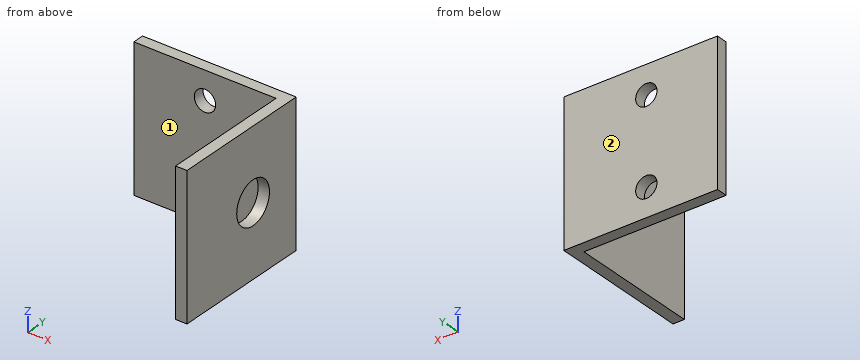
```python
from build123d import *

# Parameters (mm, degrees)
SKETCH2_W           = 20
SKETCH2_H           = 20
BOSS_EXTRUDE1_DEPTH = 1.6
SKETCH2_4_W         = 1.6
SKETCH2_4_H         = 20
BOSS_EXTRUDE2_DEPTH = 20
SKETCH3_R           = 3
CUT_EXTRUDE1_DEPTH  = 3
SKETCH4_R           = 1.5
CUT_EXTRUDE2_DEPTH  = 2


with BuildPart() as part:
    # Sketch2 → Boss-Extrude1 (new body)
    with BuildSketch(Plane(origin=(0, 0, 0), x_dir=(1, 0, 0), z_dir=(0, 1, 0))):
        Rectangle(SKETCH2_W, SKETCH2_H)
    extrude(amount=-BOSS_EXTRUDE1_DEPTH)

    # Sketch2_4 → Boss-Extrude2 (add)
    with BuildSketch(Plane(origin=(0, 0, 0), x_dir=(1, 0, 0), z_dir=(0, 1, 0))):
        with Locations((10.8, 0)):
            Rectangle(SKETCH2_4_W, SKETCH2_4_H)
    extrude(amount=-BOSS_EXTRUDE2_DEPTH)

    # Sketch3 → Cut-Extrude1 (cut)
    with BuildSketch(Plane(origin=(11.6, 0, 0), x_dir=(0, 0, -1), z_dir=(1, 0, 0))):
        with Locations((0, -7.888677581)):
            Circle(SKETCH3_R)
    extrude(amount=-CUT_EXTRUDE1_DEPTH, mode=Mode.SUBTRACT)

    # Sketch4 → Cut-Extrude2 (cut)
    with BuildSketch(Plane(origin=(0, 0, 0), x_dir=(1, 0, 0), z_dir=(0, 1, 0))):
        with Locations(Location((0, 6, 0), (0, 0, 270))):
            Circle(SKETCH4_R)
        with Locations(Location((0, -6, 0), (0, 0, 270))):
            Circle(SKETCH4_R)
    extrude(amount=-CUT_EXTRUDE2_DEPTH, mode=Mode.SUBTRACT)


solid = part.part
```
For this review, take the finished solid that the model builds, in its own axes (mm). Face numbers are marked on the shaded views. A direction names the side the tool comes from. Give positions to 0.01 mm unless a question says otherwise; leave off trailing zeros. Order: outer loops, then holes, each group sorted by start corner. A loop starts at its lowest first (then second) coordinate and runs counter-clockwise, first axis right, second up.
1) Take a section at C-C (y = -6.5). Give the boundary of the cut face in (x, z).
2) Wall thickness on line 1 (Y direction, x = -8.25, z = -4); line 2 (X direction, y = -5.75, z = 5.25); line 3 (Y direction, x = 10.4, z = 0): over which ranges is each line inside the solid? List them lowest first.
3) Take a section at A-A (z = 6). Give the boundary of the cut face in (x, y), then the cut area to 3 significant figures.
4) Take a section at D-D (z = 0). Give the boundary of the cut face in (x, y), then the cut area to 3 significant figures.
5) For the marked faces 1 and 2, list the 3-axis set-ups (+Z, -Z, +X, -X, +Y, -Y) from which the entire face can be reached by the end or side of a thin tool; tool diameter is ignored.
6) Take a section at B-B (x = 0). Give the boundary of the cut face in (y, z), then the cut area to 3 significant figures.
7) Insertion check: pin 1 (5.5 mm diameter, centred on y = -9.5, z = 2.5, fed in from -X); pin 2 (1.8 mm diameter, centred on x = 0, z = -6, fed in from -Y); pin 3 (12 mm diameter, centred on x = -6.5, z = 3.5, fed in from -Y). Each pin has a flat end and moves straight along its axis. Give the tip position at first contact, or say it passes through.
Derived:
1. outline: (10, -10) - (11.6, -10) - (11.6, -2.66) - (10, -2.66) - close; (10, 2.66) - (11.6, 2.66) - (11.6, 10) - (10, 10) - close
2. line 1: y = -1.6 to 0
2. line 2: x = 10 to 11.6
2. line 3: y = -20 to -10.89, -4.89 to 0
3. outline: (-10, -1.6) - (-1.5, -1.6) - (-1.5, 0) - (-10, 0) - close; (1.5, -1.6) - (10, -1.6) - (10, -20) - (11.6, -20) - (11.6, 0) - (1.5, 0) - close
3. area: 59.2 mm2
4. outline: (-10, -1.6) - (10, -1.6) - (10, -4.89) - (11.6, -4.89) - (11.6, 0) - (-10, 0) - close; (10, -20) - (11.6, -20) - (11.6, -10.89) - (10, -10.89) - close
4. area: 54.4 mm2
5. face 1: +Z, -Z, -X, -Y
5. face 2: +Z, -Z, +X, -X, +Y
6. outline: (-1.6, -10) - (0, -10) - (0, -7.5) - (-1.6, -7.5) - close; (-1.6, -4.5) - (0, -4.5) - (0, 4.5) - (-1.6, 4.5) - close; (-1.6, 7.5) - (0, 7.5) - (0, 10) - (-1.6, 10) - close
6. area: 22.4 mm2
7. pin 1: stops at x = 10
7. pin 2: passes through
7. pin 3: stops at y = -1.6
